Work out the finished part from the listing and answer in its coordinate system (mm). Face numbers are marked on the shaded views. A direction names the side the tool comes from. Round coordinates to 2 decimals unless told otherwise and drop trailing zeros. Order: outer loops, then holes, each group sorted by start corner. A loop starts at its lowest first (then second) coordinate and runs counter-clockwise, first axis right, second up. Notation, with made-up numbers: (7.5, -26.75) - (48.5, -26.75) arc R24 cw to (48.5, -11.75) - close; hole circle Ø11 at (50, 44.25). An arc over 180 degrees is marked (long way). Put each result on its own line as item: value.
```python
from build123d import *

# Parameters (mm, degrees)
F1_DEPTH = 45
F3_DEPTH = 15
F4_W     = 19
F4_H     = 8
F5_DEPTH = 6
F7_DEPTH = 15
F8_R     = 3
F9_R     = 5


with BuildPart() as f1:
    # F0 (on Front) → F1 (new body, symmetric)
    with BuildSketch(Plane.XZ):
        Polygon((12, -20.78461), (24, 0), (12, 20.78461), (-12, 20.78461), (-24, 0), (-12, -20.78461), align=None)
        with BuildLine():
            Line((12, 20.78461), (24, 0))
            ThreePointArc((24, 0), (20.78461, 12), (12, 20.78461))
        make_face()
        with BuildLine():
            Line((-12, 20.78461), (12, 20.78461))
            ThreePointArc((12, 20.78461), (0, 24), (-12, 20.78461))
        make_face()
        with BuildLine():
            Line((-24, 0), (-12, 20.78461))
            ThreePointArc((-12, 20.78461), (-20.78461, 12), (-24, 0))
        make_face()
    extrude(amount=F1_DEPTH, both=True)

    # F2 (on face) → F3 (join)
    with BuildSketch(Plane.XZ.offset(45)):
        Polygon((-12, -41.569219), (12, -41.569219), (24, -20.78461), (12, 0), (-12, 0), (-24, -20.78461), align=None)
        Polygon((-24, 0), (-24, -20.78461), (-18, -10.392305), align=None)
        Polygon((18, -10.392305), (24, -20.78461), (24, 0), align=None)
    extrude(amount=-F3_DEPTH)

    # F4 (on face) → F5 (cut)
    with BuildSketch(Plane(origin=(0, 0, -41.569219), x_dir=(1, 0, 0), z_dir=(0, 0, -1))):
        with Locations((0, 37.5)):
            Rectangle(F4_W, F4_H)
    extrude(amount=-F5_DEPTH, mode=Mode.SUBTRACT)

    # F6 (on face) → F7 (join)
    with BuildSketch(Plane(origin=(0, 45, 0), x_dir=(-1, 0, 0), z_dir=(0, 1, 0))):
        Polygon((5.75, -9.959292), (11.5, 0), (5.75, 9.959292), (-5.75, 9.959292), (-11.5, 0), (-5.75, -9.959292), align=None)
    extrude(amount=F7_DEPTH)

    # F8
    f8_edges = [f1.edges().sort_by_distance(p)[0] for p in [
        (9.5, -37.5, -35.569219),
        (0, -41.5, -35.569219),
        (-9.5, -37.5, -35.569219),
        (0, -33.5, -35.569219),
    ]]
    fillet(f8_edges, radius=F8_R)

    # F9
    f9_edges = [f1.edges().sort_by_distance(p)[0] for p in [
        (11.5, 52.5, 0),
        (5.75, 52.5, 9.959292),
        (-5.75, 52.5, 9.959292),
        (-11.5, 52.5, 0),
        (-5.75, 52.5, -9.959292),
        (5.75, 52.5, -9.959292),
    ]]
    fillet(f9_edges, radius=F9_R)


solid = f1.part
```
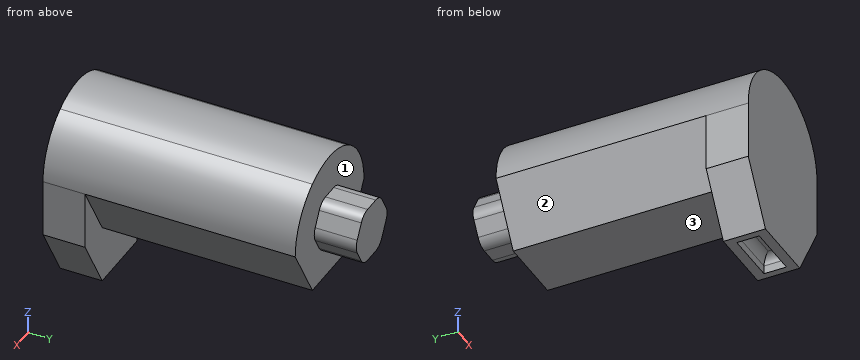
1) For the marked faces 1, 2 and 3, determine the directions among +Z, -Z, +X, -X, +Y, -Y from which every point of the face is accessible in a straight line to the end or side of a thin tool.
Findings below:
face 1: +Y
face 2: -Z, -X, +Y
face 3: -Z, +X, -X, +Y
2) A cutting plane is placed at D-D on y = -32. Write down the section's boundary in (x, z), then the cut area to 3 significant figures.
Findings below:
outline: (-24, -20.78) - (-12, -41.57) - (12, -41.57) - (24, -20.78) - (24, 0) arc R24 ccw to (12, 20.78) arc R24 ccw to (-12, 20.78) arc R24 ccw to (-24, 0) - close
area: 2,650 mm2
3) Straight lines are drawn through the part: L1, parallel to Y at x = 3, z = -13.5; L2, parallel to Y at x = 17.5, z = -21.5; L3, parallel to Z at x = -3, y = 46.5. For each, find the intervals that lie inside material, in ascending order. Write a range as from..to.
Findings below:
L1: y = -45..45
L2: y = -45..-30
L3: z = -9.96..9.96
4) Given pin 1 Ø3 at (y, z) = (45, 13.5) entering from +X; pin 2 Ø2.5 at (x, z) = (-4.5, -40.5) entering from +Y; pin 3 Ø12 at (x, y) = (-3, -0.5) entering from -Z, each flat-ended and moving along its own axis, determine where each tip first touches the part or whether it passes through.
Findings below:
pin 1: stops at x = 20.78
pin 2: stops at y = -30
pin 3: stops at z = -20.78
5) A cutting plane is placed at C-C on x = 4. Write down the section's boundary in (y, z), then the cut area to 3 significant figures.
Findings below:
outline: (-45, -41.57) - (-41.5, -41.57) - (-41.5, -38.57) arc R3 cw to (-38.5, -35.57) - (-36.5, -35.57) arc R3 cw to (-33.5, -38.57) - (-33.5, -41.57) - (-30, -41.57) - (-30, -20.78) - (45, -20.78) - (45, -9.83) - (60, -9.83) - (60, 9.83) - (45, 9.83) - (45, 23.66) - (-45, 23.66) - close
area: 4,560 mm2
6) A cutting plane is placed at A-A on y = -19.5. Write down the section's boundary in (x, z).
Findings below:
outline: (-24, 0) - (-12, -20.78) - (12, -20.78) - (24, 0) arc R24 ccw to (12, 20.78) arc R24 ccw to (-12, 20.78) arc R24 ccw to start
7) A cutting plane is placed at B-B on z = -14. Write down the section's boundary in (x, y).
Findings below:
outline: (-24, -45) - (24, -45) - (24, -30) - (15.92, -30) - (15.92, 45) - (-15.92, 45) - (-15.92, -30) - (-24, -30) - close
